```python
from build123d import *

# Parameters (mm, degrees)
F0_W     = 92.3412963748
F0_H     = 87.5617265701
F1_DEPTH = 25.4
F2_T     = -10.16
F3_R     = 5.07999


# Not quite as in the source:
# - a fillet or chamfer is up to 0.001 mm smaller than in the source, because OpenCascade refuses the exact size


with BuildPart() as f1:
    # F0 (on Top) → F1 (new body)
    with BuildSketch(Plane.XY):
        with Locations((-0.1911818981, -0.9559132159)):
            Rectangle(F0_W, F0_H)
    extrude(amount=F1_DEPTH)

    # F2
    f2_openings = [f1.faces().sort_by_distance(p)[0] for p in [
        (-0.191182, -0.955913, 25.4),
    ]]
    offset(amount=F2_T, openings=f2_openings)

    # F3 (radius 5.08 in the source; OpenCascade refuses exactly that, so slightly less here)
    f3_edges = [f1.edges().sort_by_distance(p)[0] for p in [
        (35.819466, -0.955913, 10.16),
        (-0.191182, 32.66495, 10.16),
        (-36.20183, -0.955913, 10.16),
        (-0.191182, -34.576777, 10.16),
        (45.979466, -0.955913, 25.4),
        (-0.191182, 42.82495, 25.4),
        (-46.36183, -0.955913, 25.4),
        (-0.191182, -44.736777, 25.4),
        (35.819466, -0.955913, 25.4),
        (-0.191182, -34.576777, 25.4),
        (-36.20183, -0.955913, 25.4),
        (-0.191182, 32.66495, 25.4),
    ]]
    fillet(f3_edges, radius=F3_R)


solid = f1.part
```
Geometry: final body of the model. Coordinates: model frame, mm. A direction names the side the tool comes from. Round coordinates to 2 decimals unless told otherwise and drop trailing zeros. Loops run counter-clockwise (first coordinate to the right, second up) from the corner with the lowest first, then second, coordinate; pieces in that order, holes last. Notation, with made-up numbers: (17, 86) -> (55, 86) arc R14 ccw to (55, 108) -> close; hole circle Ø7 at (26, 38.25). An arc over 180 degrees is marked (long way). Use one line per item in the form item = value.
Item 1: Cut plane D-D on z = 13. Output: boundary loops of the cut face in (x, y).
Evaluation:
outline = (-46.36, -44.74) -> (45.98, -44.74) -> (45.98, 42.82) -> (-46.36, 42.82) -> close; hole (-35.68, -34.06) -> (35.3, -34.06) -> (35.3, 32.14) -> (-35.68, 32.14) -> close
Item 2: Access query for faces 1 (the cylindrical face through (0.46, 41.38, 23.87)), 2 (the cylindrical face through (-34.753, -0.485, 11.688)). Directions: +Z, -Z, +X, -X, +Y, -Y. A direction counts if a zero-diameter tool reaches every point of the face in a straight line with its end or side. Return the directions, or none.
Evaluation:
face_1 = +Z, +X, -X, +Y
face_2 = +Z
Item 3: Contact query for a flat-ended pin moving along its axis: pin 1 Ø17 at (x, y) = (3, -0.5) entering from +Z. Output: stop coordinate, or through.
Evaluation:
pin_1 = 10.16
Item 4: Material intervals for probe 1 along X at (y, z) = (4.5, 20.25); probe 2 along Y at (x, z) = (-5, 20.5); probe 3 along Z at (x, y) = (14, -9.5), sorted ascending.
Evaluation:
probe_1 = -46.36 to -36.2, 35.82 to 45.98
probe_2 = -44.73 to -34.58, 32.67 to 42.82
probe_3 = 0 to 10.16
Item 5: Cut plane A-A on z = 18.25. Output: boundary loops of the cut face in (x, y).
Evaluation:
outline = (-46.36, -44.74) -> (45.98, -44.74) -> (45.98, 42.82) -> (-46.36, 42.82) -> close; hole (-36.2, -34.58) -> (35.82, -34.58) -> (35.82, 32.66) -> (-36.2, 32.66) -> close
Item 6: Draft query along X for faces 3 (the flat face through (-1, 42.825, 10)), 4 (the cylindrical face through (0.31, 31.22, 11.69)), 5 (the cylindrical face through (44.531, -0.343, 23.872)). Return one class per face: released by +X, released by -X, zero draft, split by the parting line, or undercut.
Evaluation:
face_3 = zero draft
face_4 = undercut
face_5 = released by +X
